from build123d import *

# Parameters (mm, degrees)
SKETCH_1_R               = 6
EXTRUDE_2_DEPTH          = 21
SKETCH_2_R               = 3
CUT_EXTRUDE_1_DEPTH      = 15
CUT_EXTRUDE_2_DEPTH      = 10
CUT_EXTRUDE_2_DEPTH_BACK = 10
SKETCH_3_R               = 3


with BuildPart() as part:
    # Sketch 1 → Extrude 2 (new body)
    with BuildSketch(Plane(origin=(0, 0, 0), x_dir=(1, 0, 0), z_dir=(0, 1, 0))):
        with Locations(Location((0, 0, 0), (0, 0, 90))):
            Circle(SKETCH_1_R)
    extrude(amount=EXTRUDE_2_DEPTH)

    # Sketch 2 → Cut-Extrude 1 (cut)
    with BuildSketch(Plane.XZ):
        with Locations(Location((0, 0, 0), (0, 0, 270))):
            Circle(SKETCH_2_R)
    extrude(amount=-CUT_EXTRUDE_1_DEPTH, mode=Mode.SUBTRACT)

    # Sketch 3 → Cut-Extrude 2 (cut, two sides: drawn at the far end of the back side and taken through both)
    with BuildSketch(Plane(origin=(0, 0, 0), x_dir=(0, 0, -1), z_dir=(1, 0, 0)).offset(-CUT_EXTRUDE_2_DEPTH_BACK)):
        with Locations(Location((0, 16.309431348, 0), (0, 0, 180))):
            Circle(SKETCH_3_R)
    extrude(amount=CUT_EXTRUDE_2_DEPTH + CUT_EXTRUDE_2_DEPTH_BACK, mode=Mode.SUBTRACT)


solid = part.part
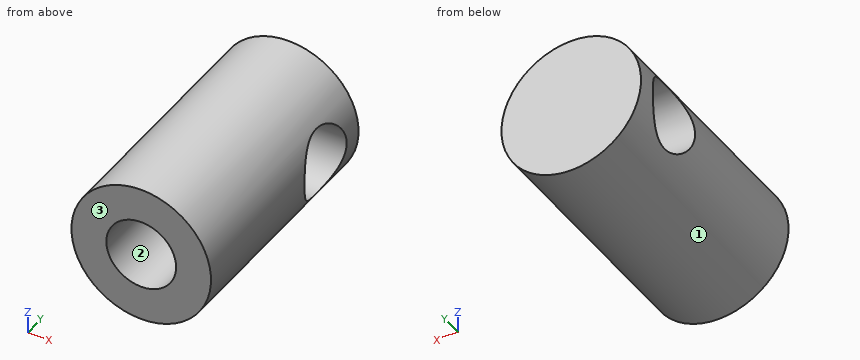
Design review of the part built by this model. Coordinates are the model's own, in mm. Face numbers are marked on the shaded views. Give positions to 0.01 mm unless a question says otherwise; leave off trailing zeros. Order: outer loops, then holes, each group sorted by start corner. A loop starts at its lowest first (then second) coordinate and runs counter-clockwise, first axis right, second up.
1. To check wall thickness, follow L1, parallel to X at y = 7.5, z = 0; L2, parallel to Z at x = 2, y = 14.25; L3, parallel to Z at x = 1, y = 12.5. State the ranges of each line that lie inside material, in increasing order.
Solution:
L1: x = -6 to -3, 3 to 6
L2: z = -5.66 to -2.24, 2.24 to 5.66
L3: z = -5.92 to -2.83, 2.83 to 5.92
2. Add section B-B, the plane x = 0. State the section outline as (y, z) points.
Solution:
outline: (0, -6) - (21, -6) - (21, 6) - (0, 6) - (0, 3) - (15, 3) - (15, 2.7) arc R3 cw (long way) to (15, -2.7) - (15, -3) - (0, -3) - close
3. Add section C-C, the plane y = 14. State the section outline as (x, z) points.
Solution:
outline: (-5.69, -1.91) arc R6 ccw to (5.69, -1.91) - (2.31, -1.91) arc R3 cw to (-2.31, -1.91) - close; (-5.69, 1.91) - (-2.31, 1.91) arc R3 cw to (2.31, 1.91) - (5.69, 1.91) arc R6 ccw to start
4. Add section A-A, the plane z = 0. State the section outline as (x, y) points.
Solution:
outline: (-6, 0) - (-3, 0) - (-3, 13.31) - (-6, 13.31) - close; (-6, 19.31) - (6, 19.31) - (6, 21) - (-6, 21) - close; (3, 0) - (6, 0) - (6, 13.31) - (3, 13.31) - close
5. For pin 1 Ø1.5 at (y, z) = (18, -2) entering from -X; pin 2 Ø2 at (y, z) = (13.5, 4) entering from -X; pin 3 Ø5 at (x, y) = (-3.5, 9) entering from -Z, all flat-tipped, find the tip position at first contact; note any pin that passes through.
Solution:
pin 1: stops at x = -5.73
pin 2: stops at x = -5.2
pin 3: stops at z = -5.92
6. Mouldability with a two-part tool opening along X and no side actions: class the marked faces 1, 2 and 3 as +X half, -X half, draft (parallel to the pull), parting line (faces both ways), or undercut.
Solution:
face 1: parting line
face 2: undercut
face 3: draft
7. Add section D-D, the plane y = 7.5. State the section outline as (x, z) points, then the cut area to 3 significant figures.
Solution:
outline: circle Ø12 at (0, 0); hole circle Ø6 at (0, 0)
area: 84.8 mm2
